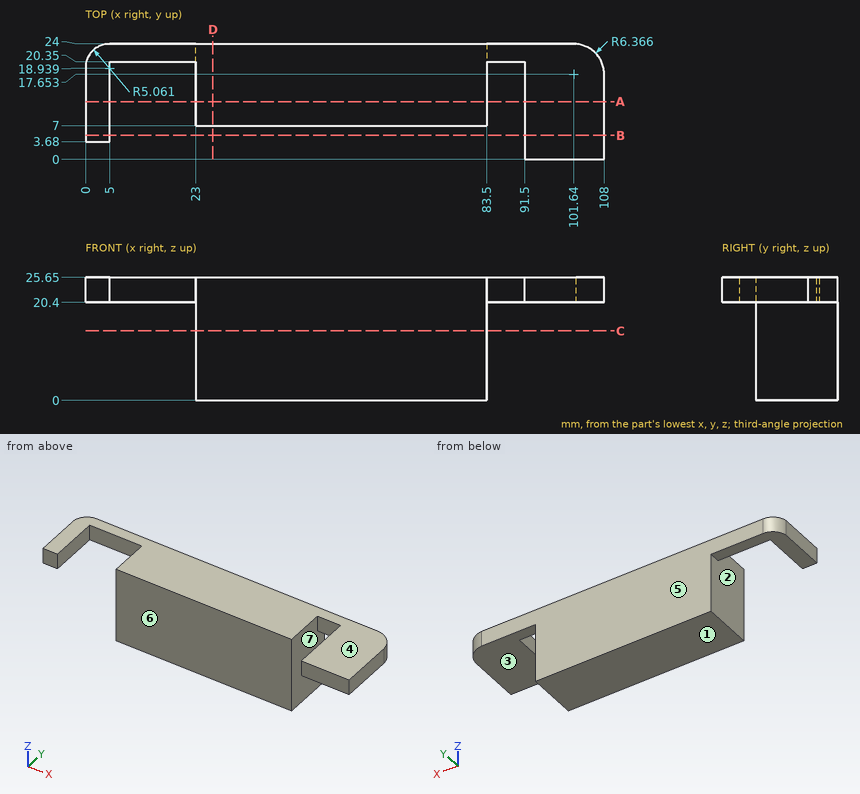
Check sheet for the drawn part. Datum: minimum x, y, z corner. Units: mm. A direction names the side the tool comes from. Round coordinates to 2 decimals unless told otherwise and drop trailing zeros. Order: outer loops, then holes, each group sorted by start corner. A loop starts at its lowest first (then second) coordinate and runs counter-clockwise, first axis right, second up. Notation, with made-up numbers: (60, -4) -> (88, -4) arc R18 cw to (88, 11) -> close; hole circle Ø11 at (15, 75.5). An arc over 180 degrees is marked (long way). Put each result on its own line as item: value.
1) Mould release check, pull along X, two halves, no side actions. Record for the marked faces 1 and 2: +X half, -X half, draft (parallel to the pull), parting line (faces both ways), or undercut.
Final values:
face 1: draft
face 2: undercut
2) Depth check by flat-ended pin: pin 1 (1.5 mm diameter, centred on y = 11, z = 9, fed in from -X); pin 2 (4 mm diameter, centred on y = 18, z = 18, fed in from +X); pin 3 (13 mm diameter, centred on x = 67.5, z = 8.5, fed in from -Y). Enter the tip coordinate at first touch or a pass-through.
Final values:
pin 1: stops at x = 23
pin 2: stops at x = 83.5
pin 3: stops at y = 7
3) Section check B-B (y = 5). Record the cut outline in (x, z), then the cut area to 3 significant figures.
Final values:
outline: (0, 20.4) -> (5, 20.4) -> (5, 25.65) -> (0, 25.65) -> close; (91.5, 20.4) -> (108, 20.4) -> (108, 25.65) -> (91.5, 25.65) -> close
area: 113 mm^2
4) Set-up check for the marked faces 3, 4, 5, 6 and 7: record each of +Z, -Z, +X, -X, +Y, -Y from which the full face is reachable in a straight line by a thin tool's end or side.
Final values:
face 3: -Z, +X, +Y, -Y
face 4: +Z, +X, -X, +Y, -Y
face 5: +Z, -Z, +X, -X, +Y
face 6: +Z, -Z, -Y
face 7: -Z, -Y
5) Material ranges on line 1 (X direction, y = 13, z = 22); line 2 (Y direction, x = 75.5, z = 18.25); line 3 (Z direction, x = 98, y = 17.5), recorded low to high.
Final values:
line 1: x = 0 to 5, 23 to 83.5, 91.5 to 108
line 2: y = 7 to 24
line 3: z = 20.4 to 25.65
6) Section check A-A (y = 12). Record the cut outline in (x, z), then the cut area to 3 significant figures.
Final values:
outline: (0, 20.4) -> (5, 20.4) -> (5, 25.65) -> (0, 25.65) -> close; (23, 0) -> (83.5, 0) -> (83.5, 25.65) -> (23, 25.65) -> close; (91.5, 20.4) -> (108, 20.4) -> (108, 25.65) -> (91.5, 25.65) -> close
area: 1,660 mm^2
7) Section check D-D (x = 26.5). Record the cut outline in (y, z), then the cut area to 3 significant figures.
Final values:
outline: (7, 0) -> (24, 0) -> (24, 25.65) -> (7, 25.65) -> close
area: 436 mm^2
8) Section check C-C (z = 14.5). Record the cut outline in (x, y), then the cut area to 3 significant figures.
Final values:
outline: (23, 7) -> (83.5, 7) -> (83.5, 24) -> (23, 24) -> close
area: 1,030 mm^2
